Design review of the part built by this model. Coordinates are the model's own, in mm. Round coordinates to 2 decimals unless told otherwise and drop trailing zeros. Write each loop counter-clockwise with the first axis right and the second up, starting at its lowest first coordinate (ties: lowest second). Pieces come first, ordered by that corner, then holes. Notation, with made-up numbers: M 0.25,5.5 L 14.25,5.5 A21 ccw 14.25,32.5 Z; hole C -6,29 d7. An arc over 180 degrees is marked long. Use CSV: the item, a comma, the result in double quotes.
from build123d import *

# Parameters (mm, degrees)
SKETCH_1_R          = 4.5
SKETCH_1_R_2        = 5
SKETCH_1_R_3        = 2
EXTRUDE_1_DEPTH     = 3
SKETCH_2_R          = 1.5
CUT_EXTRUDE_1_DEPTH = 41.317490001


with BuildPart() as part:
    # 草图1 → 凸台-拉伸1 (new body)
    # profile 1 of 3: a face of its own
    with BuildSketch(Plane(origin=(0, 0, 0), x_dir=(1, 0, 0), z_dir=(0, 1, 0))):
        with BuildLine():
            ThreePointArc((7.5, 32), (0, 39.5), (-7.5, 32))
            Line((-7.5, 32), (-7.409002669, 30.835234166))
            ThreePointArc((-7.409002669, 30.835234166), (0, 24.5), (7.409002669, 30.835234166))
            Line((7.409002669, 30.835234166), (7.5, 32))
        make_face()
        with Locations(Location((0, 32, 0), (0, 0, 270))):
            Circle(SKETCH_1_R, mode=Mode.SUBTRACT)
    # profile 2 of 3: a face of its own
    with BuildSketch(Plane(origin=(0, 0, 0), x_dir=(1, 0, 0), z_dir=(0, 1, 0))):
        Circle(SKETCH_1_R_2)
        with Locations(Location((0, 0, 0), (0, 0, 270))):
            Circle(SKETCH_1_R_3, mode=Mode.SUBTRACT)
    # profile 3 of 3: a face of its own
    with BuildSketch(Plane(origin=(0, 0, 0), x_dir=(1, 0, 0), z_dir=(0, 1, 0))):
        with BuildLine():
            ThreePointArc((7.409002669, 30.835234166), (0, 24.5), (-7.409002669, 30.835234166))
            Line((-7.409002669, 30.835234166), (-5, 0))
            ThreePointArc((-5, 0), (0, 5), (5, 0))
            Line((5, 0), (7.409002669, 30.835234166))
        make_face()
    extrude(amount=EXTRUDE_1_DEPTH)

    # 草图2 → 切除-拉伸1 (cut, through all)
    with BuildSketch(Plane(origin=(0, 3, 0), x_dir=(1, 0, 0), z_dir=(0, 1, 0))):
        with Locations(Location((0, 16, 0), (0, 0, 270))):
            Circle(SKETCH_2_R)
    extrude(amount=-CUT_EXTRUDE_1_DEPTH, mode=Mode.SUBTRACT)


solid = part.part
1) Add section A-A on z = -16. Write out the cut boundary in (x, y), then the cut area to 3 significant figures.
Answers:
outline,"M -6.25,0 L -1.5,0 L -1.5,3 L -6.25,3 Z; M 1.5,0 L 6.25,0 L 6.25,3 L 1.5,3 Z"
area,"28.5 mm²"
2) For pin 1 Ø1 at (y, z) = (0.5, -27.5) entering from +X, flat-tipped, find the tip position at first contact; note if it passes through.
Answers:
pin 1,"x = 7.19"
3) The part is to be moulded in two halves that separate along X. For faces 1 (the face through (0.07, 1.52, -17.5)), 2 (the face through (-2, 1, 0)), 3 (the face through (0, 0, -18)), 4 (the face through (0, 1, 5)), say which applies: released by +X, released by -X, zero draft, split by the parting line, or undercut.
Answers:
face 1,"undercut"
face 2,"undercut"
face 3,"zero draft"
face 4,"split by the parting line"
4) Add section C-C on x = -2.5. Write out the cut boundary in (y, z).
Answers:
outline,"M 0,-39.07 L 3,-39.07 L 3,-35.74 L 0,-35.74 Z; M 0,-28.26 L 3,-28.26 L 3,4.33 L 0,4.33 Z"
5) Add section D-D on x = -0.5. Write out the cut boundary in (y, z), then the cut area to 3 significant figures.
Answers:
outline,"M 0,-39.48 L 3,-39.48 L 3,-36.47 L 0,-36.47 Z; M 0,-27.53 L 3,-27.53 L 3,-17.41 L 0,-17.41 Z; M 0,-14.59 L 3,-14.59 L 3,-1.94 L 0,-1.94 Z; M 0,1.94 L 3,1.94 L 3,4.97 L 0,4.97 Z"
area,"86.4 mm²"
6) Wall thickness on line 1 along X through (y, z) = (1.9, 0); line 2 along X through (y, z) = (2.3, -32); line 3 along Z through (x, y) = (-3.5, 0.45): over which ranges is each line inside the solid? List them lowest first. Write a range as [from, to].
Answers:
line 1,"[-5, -2], [2, 5]"
line 2,"[-7.5, -4.5], [4.5, 7.5]"
line 3,"[-38.63, -34.83], [-29.17, 3.57]"
7) Add section B-B on y = 2.5. Write out the cut boundary in (x, z).
Answers:
outline,"M -7.5,-32 A7.5 ccw 7.5,-32 L 5,0 A5 ccw -5,0 Z; hole C 0,-32 d9; hole C 0,0 d4; hole C 0,-16 d3"
